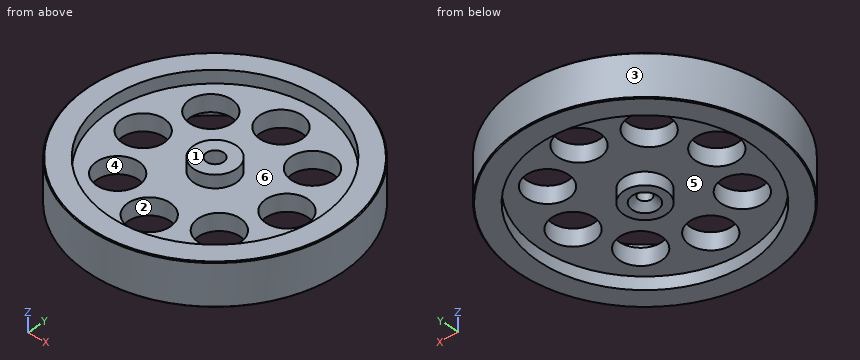
```python
from build123d import *

# Parameters (mm, degrees)
SKETCH1_R               = 30
BOSS_EXTRUDE1_DEPTH     = 5
SKETCH2_R               = 25
CUT_EXTRUDE1_DEPTH      = 3
CUT_EXTRUDE2_DEPTH      = 44
CUT_EXTRUDE2_DEPTH_BACK = 44
SKETCH3_R               = 5
SKETCH4_R               = 5
BOSS_EXTRUDE2_DEPTH     = 3
CHAMFER1_SIZE           = 0.2


with BuildPart() as part:
    # Sketch1 → Boss-Extrude1 (new, symmetric)
    with BuildSketch(Plane.XY):
        Circle(SKETCH1_R)
    extrude(amount=BOSS_EXTRUDE1_DEPTH, both=True)

    # Sketch2 → Cut-Extrude1 (cut)
    with BuildSketch(Plane.XY.offset(5)):
        Circle(SKETCH2_R)
    cut_extrude1 = extrude(amount=-CUT_EXTRUDE1_DEPTH, mode=Mode.SUBTRACT)

    # Mirror1: Cut-Extrude1 across plane
    add(cut_extrude1.mirror(Plane.XY), mode=Mode.SUBTRACT)

    # Sketch3 → Cut-Extrude2 (cut, two sides: drawn at the far end of the back side and taken through both)
    with BuildSketch(Plane.XY.offset(2).offset(-CUT_EXTRUDE2_DEPTH_BACK)):
        with Locations((0, 17)):
            Circle(SKETCH3_R)
        with Locations((12.02081528, 12.02081528)):
            Circle(SKETCH3_R)
        with Locations((17, 0)):
            Circle(SKETCH3_R)
        with Locations((12.02081528, -12.02081528)):
            Circle(SKETCH3_R)
        with Locations((0, -17)):
            Circle(SKETCH3_R)
        with Locations((-12.02081528, -12.02081528)):
            Circle(SKETCH3_R)
        with Locations((-17, 0)):
            Circle(SKETCH3_R)
        with Locations((-12.02081528, 12.02081528)):
            Circle(SKETCH3_R)
    extrude(amount=CUT_EXTRUDE2_DEPTH + CUT_EXTRUDE2_DEPTH_BACK, mode=Mode.SUBTRACT)

    # Sketch4 → Boss-Extrude2 (add)
    with BuildSketch(Plane.XY.offset(2)):
        Circle(SKETCH4_R)
    boss_extrude2 = extrude(amount=BOSS_EXTRUDE2_DEPTH)

    # Mirror2: Boss-Extrude2 across plane
    add(boss_extrude2.mirror(Plane.XY))

    # Sketch5 → Cut-Revolve1 (revolve, cut)
    with BuildSketch(Plane(origin=(0, 0, 0), x_dir=(0, 0, -1), z_dir=(1, 0, 0)), mode=Mode.PRIVATE) as cut_revolve1_sk:
        Polygon((-5, 0), (5, 0), (5, 3), (3.5, 1.5), (1, 1.5), (1, 2), (-5, 2), align=None)
    revolve(cut_revolve1_sk.sketch.rotate(Axis((0, 0, 5), (0, 0, -1)), 90), axis=Axis((0, 0, 5), (0, 0, -1)), mode=Mode.SUBTRACT)

    # Chamfer1
    chamfer1_edges = [part.edges().sort_by_distance(p)[0] for p in [
        (-30, 0, -5),
        (-30, 0, 5),
    ]]
    chamfer(chamfer1_edges, length=CHAMFER1_SIZE)


solid = part.part
```
Source: CAD feature listing. Evaluate the final solid. Frame: model axes, mm. Face numbers are marked on the shaded views. A direction names the side the tool comes from. Coordinates: 2 decimals unless noted, no trailing zeros. One line per item, written item: value.
1) Reachability of the marked faces 4, 5 and 6 from +Z, -Z, +X, -X, +Y, -Y: full face, straight path, thin tool, end or side. Return the list, or none.
Computed values:
face 4: +Z, -Z
face 5: -Z
face 6: +Z
2) Cut plane A-A on x = 0. State how many separate pieces and enclosed holes the cut face has, plus the area to 3 significant figures.
Computed values:
separate pieces: 4
enclosed holes: 0
area: 242 mm^2
3) Contact query for flat-ended pins moving along their axis: pin 1 (4 mm diameter, centred on x = -3, z = 0, fed in from +Y); pin 2 (8 mm diameter, centred on x = 12.02, y = 12.02, fed in from +Z); pin 3 (3.5 mm diameter, centred on x = 0, y = 0, fed in from +Z); pin 4 (5 mm diameter, centred on x = 0, y = 0, fed in from -Z). Output: stop coordinate, or through.
Computed values:
pin 1: stops at y = 29.98
pin 2: passes through
pin 3: stops at z = -1
pin 4: stops at z = -4.5
4) Ray query, line 1 (Y direction, x = 0, z = 0.6); line 2 (X direction, y = -16, z = 1.25); line 3 (X direction, y = 2, z = -4.5). Return the intervals inside material, ascending. Write a range as [from, to].
Computed values:
line 1: y = [-30, -22], [-12, -2], [2, 12], [22, 30]
line 2: x = [-25.38, -15.05], [-8.99, -4.9], [4.9, 8.99], [15.05, 25.38]
line 3: x = [-29.93, -24.92], [-4.58, -1.5], [1.5, 4.58], [24.92, 29.93]
5) Mould query, pull axis Y, two halves, no side actions, for the marked faces 1, 2 and 3. Classes: released by +Y, released by -Y, zero draft, split by the parting line, or undercut.
Computed values:
face 1: zero draft
face 2: undercut
face 3: split by the parting line
